Part model, mm, in its own coordinate system. A direction names the side the tool comes from. Round coordinates to 2 decimals unless told otherwise and drop trailing zeros. Loops run counter-clockwise (first coordinate to the right, second up) from the corner with the lowest first, then second, coordinate; pieces in that order, holes last.
1) 3-axis set-ups, long thin cutter, end or side, ignore diameter. For faces 4 (the flat face through (19, 78, 2)), 5 (the flat face through (54, -16, 2)): which of +Z, -Z, +X, -X, +Y, -Y reach the whole face in a straight line?
2) Probe line 1 (X direction, y = 84, z = 2.05); line 2 (Y direction, x = 36, z = 1.65); line 3 (Y direction, x = 106.7, z = 1.3). List the from-to ranges inside material, lowest first.
3) Band-saw the part on D-D, the plane x = 16. Write the cut outline in (y, z), then the cut area to 3 significant figures.
4) Band-saw the part on A-A, the plane x = 106.7. Write the cut outline in (y, z), then the cut area to 3 significant figures.
5) Mould opens along X. For faces 1 (the flat face through (54, 37, 3)), 2 (the cylindrical face through (34.8, -5.9, 1.5)), 3 (the flat face through (0, 37, 1)) say: +X half, -X half, draft (parallel to the pull), parting line (faces both ways), or undercut.
6) Band-saw the part on B-B, the plane y = 84. Write the cut outline in (x, z), then the cut area to 3 significant figures.
7) Band-saw the part on C-C, the plane z = 0.5. State how many separate pieces and enclosed holes the cut face has, then the cut area to 3 significant figures.
from build123d import *

# Parameters (mm, degrees)
CROQUIS1_W                   = 110
CROQUIS1_H                   = 92
SALIENTE_EXTRUIR1_DEPTH      = 3
CROQUIS7_W                   = 110
CROQUIS7_H                   = 3
SALIENTE_EXTRUIR2_DEPTH      = 6
CROQUIS8_W                   = 110
CROQUIS8_H                   = 3
SALIENTE_EXTRUIR3_DEPTH      = 6
TALADRO_DE_MARGEN_PARA_M31_D = 3.2
CORTAR_EXTRUIR2_REACH        = 142.901
CROQUIS13_R                  = 1.5
CORTAR_EXTRUIR3_REACH        = 142.901
CROQUIS14_W                  = 12
CROQUIS14_H                  = 84


with BuildPart() as part:
    # Croquis1 → Saliente-Extruir1 (new body)
    with BuildSketch(Plane.XY):
        with Locations((55, 36)):
            Rectangle(CROQUIS1_W, CROQUIS1_H)
    extrude(amount=SALIENTE_EXTRUIR1_DEPTH)

    # Croquis7 → Saliente-Extruir2 (add)
    with BuildSketch(Plane(origin=(0, 82, 0), x_dir=(1, 0, 0), z_dir=(0, 1, 0))):
        with Locations((55, -1.5)):
            Rectangle(CROQUIS7_W, CROQUIS7_H)
    extrude(amount=SALIENTE_EXTRUIR2_DEPTH)

    # Croquis8 → Saliente-Extruir3 (add)
    with BuildSketch(Plane.XZ.offset(10)):
        with Locations((55, 1.5)):
            Rectangle(CROQUIS8_W, CROQUIS8_H)
    extrude(amount=SALIENTE_EXTRUIR3_DEPTH)

    # Taladro de margen para M31 (through all)
    with Locations(Plane(origin=(3.3, 84, 3), x_dir=(1, 0, 0), z_dir=(0, 0, 1))):
        with Locations((0, 0), (0, -96), (103.4, -96), (103.4, 0)):
            Hole(TALADRO_DE_MARGEN_PARA_M31_D / 2)

    # Croquis13 → Cortar-Extruir2 (cut, up to next)
    with BuildSketch(Plane.XY.offset(3), mode=Mode.PRIVATE) as cortar_extruir2_sk1:
        with Locations((36, 53)):
            Circle(CROQUIS13_R)
    cortar_extruir2_tool1 = extrude(cortar_extruir2_sk1.sketch, amount=-CORTAR_EXTRUIR2_REACH, mode=Mode.PRIVATE) & part.part
    # Croquis13 → Cortar-Extruir2 (cut, up to next)
    with BuildSketch(Plane.XY.offset(3), mode=Mode.PRIVATE) as cortar_extruir2_sk2:
        with Locations((85, 53)):
            Circle(CROQUIS13_R)
    cortar_extruir2_tool2 = extrude(cortar_extruir2_sk2.sketch, amount=-CORTAR_EXTRUIR2_REACH, mode=Mode.PRIVATE) & part.part
    # Croquis13 → Cortar-Extruir2 (cut, up to next)
    with BuildSketch(Plane.XY.offset(3), mode=Mode.PRIVATE) as cortar_extruir2_sk3:
        with Locations((36, -5)):
            Circle(CROQUIS13_R)
    cortar_extruir2_tool3 = extrude(cortar_extruir2_sk3.sketch, amount=-CORTAR_EXTRUIR2_REACH, mode=Mode.PRIVATE) & part.part
    # Croquis13 → Cortar-Extruir2 (cut, up to next)
    with BuildSketch(Plane.XY.offset(3), mode=Mode.PRIVATE) as cortar_extruir2_sk4:
        with Locations((85, -5)):
            Circle(CROQUIS13_R)
    cortar_extruir2_tool4 = extrude(cortar_extruir2_sk4.sketch, amount=-CORTAR_EXTRUIR2_REACH, mode=Mode.PRIVATE) & part.part
    add(cortar_extruir2_tool1.solids().sort_by_distance((36, 53, 3))[0], mode=Mode.SUBTRACT)
    add(cortar_extruir2_tool2.solids().sort_by_distance((85, 53, 3))[0], mode=Mode.SUBTRACT)
    add(cortar_extruir2_tool3.solids().sort_by_distance((36, -5, 3))[0], mode=Mode.SUBTRACT)
    add(cortar_extruir2_tool4.solids().sort_by_distance((85, -5, 3))[0], mode=Mode.SUBTRACT)

    # Croquis14 → Cortar-Extruir3 (cut, up to next)
    with BuildSketch(Plane.XY.offset(3), mode=Mode.PRIVATE) as cortar_extruir3_sk1:
        with Locations((19, 36)):
            Rectangle(CROQUIS14_W, CROQUIS14_H)
    cortar_extruir3_tool1 = extrude(cortar_extruir3_sk1.sketch, amount=-CORTAR_EXTRUIR3_REACH, mode=Mode.PRIVATE) & part.part
    add(cortar_extruir3_tool1.solids().sort_by_distance((19, 36, 3))[0], mode=Mode.SUBTRACT)


solid = part.part
Reported:
1. face 4: +Z, -Z
1. face 5: +Z, -Z, +X, -X, -Y
2. line 1: x = 0 to 1.7, 4.9 to 105.1, 108.3 to 110
2. line 2: y = -16 to -6.5, -3.5 to 51.5, 54.5 to 88
2. line 3: y = -16 to -13.6, -10.4 to 82.4, 85.6 to 88
3. outline: (-16, 0) - (-6, 0) - (-6, 3) - (-16, 3) - close; (78, 0) - (88, 0) - (88, 3) - (78, 3) - close
3. area: 60.0 mm2
4. outline: (-16, 0) - (-13.6, 0) - (-13.6, 3) - (-16, 3) - close; (-10.4, 0) - (82.4, 0) - (82.4, 3) - (-10.4, 3) - close; (85.6, 0) - (88, 0) - (88, 3) - (85.6, 3) - close
4. area: 293 mm2
5. face 1: draft
5. face 2: undercut
5. face 3: -X half
6. outline: (0, 0) - (1.7, 0) - (1.7, 3) - (0, 3) - close; (4.9, 0) - (105.1, 0) - (105.1, 3) - (4.9, 3) - close; (108.3, 0) - (110, 0) - (110, 3) - (108.3, 3) - close
6. area: 311 mm2
7. separate pieces: 1
7. enclosed holes: 9
7. area: 10,400 mm2
